The model under review builds one solid part; all positions refer to its coordinate system, in mm. A direction names the side the tool comes from. Coordinates: 2 decimals unless noted, no trailing zeros. Write each loop counter-clockwise with the first axis right and the second up, starting at its lowest first coordinate (ties: lowest second). Pieces come first, ordered by that corner, then holes.
1) Mouldability with a two-part tool opening along Y and no side actions: class faces 1 (the cylindrical face through (-38.65, 59.37, 10.12)), 2 (the flat face through (66.234, -37.681, 6.261)), 3 (the flat face through (-66.234, 37.681, 6.261)) as released by +Y, released by -Y, zero draft, split by the parting line, or undercut.
2) For line 1 (Y direction, x = 44.5, z = 7.5); line 2 (X direction, y = 36.5, z = 12); line 3 (X direction, y = -15.5, z = 10.5), list the stretches that pass through material, from the lowest coordinate up.
3) Add section B-B, the plane y = -64.5. State the section outline as (x, z) points.
4) For P1, Ø5, axis at y = 50, z = 1.5, coming from the +X side; P2, Ø3, axis at y = -30, z = 10.5, coming from the +X side; P3, Ø1, axis at x = 50, z = 2, coming from the -Y side; P4, Ø2, axis at x = 68, y = 39, coming from the -Z side, all flat-tipped, find the tip position at first contact; note any pin that passes through.
5) Machinability: for faces 4 (the cylindrical face through (45.766, -53.426, 10.124)), 5 (the flat face through (-1, 1, 12.7)), which of the approach directions +Z, -Z, +X, -X, +Y, -Y give a long, thin tool a straight path to every point of the face, cutting with its end or side? Answer none if there is none.
6) Add section C-C, the plane x = -52. State the section outline as (y, z) points.
7) Add section A-A, the plane z = 10.25. State the section outline as (x, y) points.
from build123d import *

# Parameters (mm, degrees)
F1_DEPTH = 12.7
F3_D     = 5.9944
F3_DEPTH = 5.08
F3_TIP   = 1.8008994473


with BuildPart() as f1:
    # F0 (on Top) → F1 (new body)
    with BuildSketch(Plane.XY):
        Polygon((45.0902102752, -75.5565545624), (87.979000811, 1.2709902791), (42.8887905359, 76.8275448415), (-45.0902102752, 75.5565545624), (-87.979000811, -1.2709902791), (-42.8887905359, -76.8275448415), align=None)
    extrude(amount=F1_DEPTH)

    # F3
    with Locations(Plane.XY.offset(12.7)):
        with Locations((-39.0446968377, 56.39789626), (43.9692549407, 56.39789626), (-39.0446968377, -56.39789626), (45.3762710094, -56.39789626)):
            Hole(F3_D / 2, depth=F3_DEPTH)
            with Locations((0, 0, -(F3_DEPTH + F3_TIP / 2))):  # 118° drill point
                Cone(0, F3_D / 2, F3_TIP, mode=Mode.SUBTRACT)


solid = f1.part
Geometry results:
1. face 1: undercut
1. face 2: released by -Y
1. face 3: released by +Y
2. line 1: y = -75.57 to -59.05, -53.74 to 53.65, 59.14 to 74.13
2. line 2: x = -66.89 to 66.96
2. line 3: x = -79.49 to 78.62
3. outline: (-50.25, 0) - (51.26, 0) - (51.26, 12.7) - (-50.25, 12.7) - close
4. P1: stops at x = 60.39
4. P2: stops at x = 71.36
4. P3: stops at y = -67.66
4. P4: passes through
5. face 4: +Z
5. face 5: +Z, +X, -X, +Y, -Y
6. outline: (-61.56, 0) - (63.18, 0) - (63.18, 12.7) - (-61.56, 12.7) - close
7. outline: (-87.98, -1.27) - (-42.89, -76.83) - (45.09, -75.56) - (87.98, 1.27) - (42.89, 76.83) - (-45.09, 75.56) - close; hole circle Ø5.99 at (-39.04, -56.4); hole circle Ø5.99 at (-39.04, 56.4); hole circle Ø5.99 at (43.97, 56.4); hole circle Ø5.99 at (45.38, -56.4)
